from build123d import *

# Parameters (mm, degrees)
EXTRUDE1_DEPTH     = 3.36042
CIRPATTERN1_COUNT  = 2
CIRPATTERN1_ANGLE  = 90
SKETCH4_R          = 2.1209
CUT_EXTRUDE1_DEPTH = 24.4950001


with BuildPart() as part:
    # Sketch1 → Revolve1 (revolve)
    with BuildSketch(Plane.XY):
        Polygon((23.495, 2.1209), (23.495, 2.651125), (22.437725, 2.651125), (15.0368, 4.0005), (15.0368, 3.2004), (6.1087, 3.2004), (6.1087, 4.8006), (3.7592, 4.8006), (3.7592, 3.84048), (0, 3.84048), (0, 2.1209), align=None)
    revolve(axis=Axis((0, 0, 0), (1, 0, 0)))

    # Sketch2 → Revolve2 (revolve)
    with BuildSketch(Plane.XY):
        with BuildLine():
            Line((7.7089, 3.2004), (6.1087, 3.2004))
            Line((6.1087, 3.2004), (6.1087, 4.8006))
            ThreePointArc((6.1087, 4.8006), (6.577387729, 3.669087729), (7.7089, 3.2004))
        make_face()
        with BuildLine():
            Line((3.7592, 4.8006), (3.7592, 3.84048))
            Line((3.7592, 3.84048), (2.79908, 3.84048))
            ThreePointArc((2.79908, 3.84048), (3.477987363, 4.121692637), (3.7592, 4.8006))
        make_face()
    revolve(axis=Axis((0, 0, 0), (1, 0, 0)))

    # Sketch3 → Extrude1 (add, symmetric)
    with BuildSketch(Plane(origin=(0, 0, 0), x_dir=(-1, 0, 0), z_dir=(0, 0.707106781, 0.707106781))):
        with BuildLine():
            Line((-9.5754825, 0.5286375), (-13.1702175, 0.5286375))
            ThreePointArc((-13.1702175, 0.5286375), (-13.698855, 0), (-13.1702175, -0.5286375))
            Line((-13.1702175, -0.5286375), (-9.5754825, -0.5286375))
            ThreePointArc((-9.5754825, -0.5286375), (-9.046845, 0), (-9.5754825, 0.5286375))
        make_face()
    extrude1 = extrude(amount=EXTRUDE1_DEPTH, both=True)

    # CirPattern1: Extrude1 ×2 about axis
    cirpattern1_axis = Axis((0, 0, 0), (1, 0, 0))
    for i in range(1, CIRPATTERN1_COUNT):
        add(extrude1.rotate(cirpattern1_axis, i * CIRPATTERN1_ANGLE / (CIRPATTERN1_COUNT - 1)))

    # Sketch4 → Cut-Extrude1 (cut, through all)
    with BuildSketch(Plane(origin=(23.495, 0, 0), x_dir=(0, 0, -1), z_dir=(1, 0, 0))):
        Circle(SKETCH4_R)
    extrude(amount=-CUT_EXTRUDE1_DEPTH, mode=Mode.SUBTRACT)

    # Mirror1: part across plane


with BuildPart() as part_1:
    add(part.part)
    add(part.part.mirror(Plane(origin=(0, 0, 0), x_dir=(0, 0, 1), z_dir=(1, 0, 0))))


solid = part_1.part
Verification items for the finished model (mm, model axes). A direction names the side the tool comes from. Coordinates: 2 decimals unless noted, no trailing zeros. Answer as a JSON object with one key per item and string values. Group by question number.
Item 1: Scan lines: probe 1 along Z at (x, y) = (15, 0); probe 2 along Z at (x, y) = (-5.5, 0); probe 3 along Y at (x, z) = (-15.5, 1.5). Record each from-to range of solid material in increasing order.
Item 2: Depth check by flat-ended pin: pin 1 (5.5 mm diameter, centred on y = 0, z = 0, fed in from -X) (3 decimals); pin 2 (1 mm diameter, centred on x = -1, y = 3, fed in from +Z); pin 3 (2.5 mm diameter, centred on y = 0, z = 0, fed in from +X). Enter the tip coordinate at first touch or a pass-through.
Item 3: Tool access check on faces 1 (the conical face through (19.51, -0.69, -3.11)), 2 (the cylindrical face through (-22.959, 2.529, 0.796)), 3 (the cylindrical face through (11.322, 3.053, 0.961)). Record the directions out of +Z, -Z, +X, -X, +Y, -Y that give a thin tool (end or side, any length) a straight path to the whole face; none if there is none.
Evaluation:
{
 "1": {"probe 1": "z = -3.2 to -2.12, 2.12 to 3.2", "probe 2": "z = -4.8 to -2.12, 2.12 to 4.8", "probe 3": "y = -3.62 to -1.5, 1.5 to 3.62"},
 "2": {"pin 1": "stops at x = -23.495", "pin 2": "stops at z = 2.92", "pin 3": "passes through"},
 "3": {"face 1": "+X", "face 2": "-X", "face 3": "none"}
}
